Check sheet for the modelled part. Datum: model origin and axes. Units: mm. A direction names the side the tool comes from. Give positions to 0.01 mm unless a question says otherwise; leave off trailing zeros. Loops run counter-clockwise (first coordinate to the right, second up) from the corner with the lowest first, then second, coordinate; pieces in that order, holes last. Notation, with made-up numbers: M 54,-33 L 84,-33 A27 ccw 84,-8 Z; hole C -20,-33 d5. An arc over 180 degrees is marked long. Put each result on its own line as item: value. Start each with the question number.
```python
from build123d import *

# Parameters (mm, degrees)
SKETCH_1_R               = 23.95
EXTRUDE_1_DEPTH          = 1.25
SKETCH_2_W               = 2.45
SKETCH_2_H               = 4.95
CUT_EXTRUDE_1_DEPTH      = 3.5
SKETCH_3_R               = 0.75
CUT_EXTRUDE_2_DEPTH      = 3.5
SKETCH_4_R               = 1.55
CUT_EXTRUDE_3_DEPTH      = 3.5
PATTERN_CIRCULAR_1_COUNT = 5


with BuildPart() as part:
    # 草图1 → 凸台-拉伸1 (new body, symmetric)
    with BuildSketch(Plane.XY):
        with BuildLine():
            ThreePointArc((-15.121874884, 32.67), (-21.160269083, 29.124611797), (-26.398100061, 24.477342853))
            ThreePointArc((-26.398100061, 24.477342853), (-25.67852594, 8.343458848), (-35.743932713, -4.286172441))
            ThreePointArc((-35.743932713, -4.286172441), (-34.238034587, -11.124611797), (-31.43679796, -17.542170163))
            ThreePointArc((-31.43679796, -17.542170163), (-15.870201812, -21.843458848), (-6.969090425, -35.31900025))
            ThreePointArc((-6.969090425, -35.31900025), (0, -36), (6.969090425, -35.31900025))
            ThreePointArc((6.969090425, -35.31900025), (15.870201812, -21.843458848), (31.43679796, -17.542170163))
            ThreePointArc((31.43679796, -17.542170163), (34.238034587, -11.124611797), (35.743932713, -4.286172441))
            ThreePointArc((35.743932713, -4.286172441), (25.67852594, 8.343458848), (26.398100061, 24.477342853))
            ThreePointArc((26.398100061, 24.477342853), (21.160269083, 29.124611797), (15.121874884, 32.67))
            ThreePointArc((15.121874884, 32.67), (0, 27), (-15.121874884, 32.67))
        make_face()
        Circle(SKETCH_1_R, mode=Mode.SUBTRACT)
    extrude(amount=EXTRUDE_1_DEPTH, both=True)

    # 草图2 → 切除-拉伸1 (cut, through all)
    with BuildSketch(Plane.XY.offset(1.25)):
        with Locations((0, -31)):
            Rectangle(SKETCH_2_W, SKETCH_2_H)
    cut_extrude_1 = extrude(amount=-CUT_EXTRUDE_1_DEPTH, mode=Mode.SUBTRACT)

    # 草图3 → 切除-拉伸2 (cut, through all)
    with BuildSketch(Plane.XY.offset(1.25)):
        with Locations((-1.225, -29.275)):
            Circle(SKETCH_3_R)
        with Locations((1.225, -29.275)):
            Circle(SKETCH_3_R)
        with Locations((-1.225, -32.725)):
            Circle(SKETCH_3_R)
        with Locations((1.225, -32.725)):
            Circle(SKETCH_3_R)
    cut_extrude_2 = extrude(amount=-CUT_EXTRUDE_2_DEPTH, mode=Mode.SUBTRACT)

    # 草图4 → 切除-拉伸3 (cut, through all)
    with BuildSketch(Plane.XY.offset(1.25)):
        with Locations((-4.725, -30)):
            Circle(SKETCH_4_R)
        with Locations((4.725, -30)):
            Circle(SKETCH_4_R)
    cut_extrude_3 = extrude(amount=-CUT_EXTRUDE_3_DEPTH, mode=Mode.SUBTRACT)

    # 阵列(圆周)1: 切除-拉伸1, 切除-拉伸2, 切除-拉伸3 ×5 about axis
    pattern_circular_1_axis = Axis((0, 0, 0), (0, 0, 1))
    for i in range(1, PATTERN_CIRCULAR_1_COUNT):
        add(cut_extrude_1.rotate(pattern_circular_1_axis, i * 360 / PATTERN_CIRCULAR_1_COUNT), mode=Mode.SUBTRACT)
        add(cut_extrude_2.rotate(pattern_circular_1_axis, i * 360 / PATTERN_CIRCULAR_1_COUNT), mode=Mode.SUBTRACT)
        add(cut_extrude_3.rotate(pattern_circular_1_axis, i * 360 / PATTERN_CIRCULAR_1_COUNT), mode=Mode.SUBTRACT)


solid = part.part
```
Q1. Section check C-C, the plane z = 0.8. Give the number of separate pieces and of enclosed holes in the cut face, then the cut area to 3 significant figures.
Q2. Section check B-B, the plane y = 0. Record the cut outline in (x, z), then the cut area to 3 significant figures.
Q3. Thickness scan on line 1 along X through (y, z) = (-12.5, -0.5); line 2 along X through (y, z) = (26, -1.05); line 3 along Y through (x, z) = (13.5, 1.05). Record the ranges inside material, lowest first. Write a range as [from, to].
Q4. Section check A-A, the plane x = 0. Record the cut outline in (y, z) (3 decimals).
Q5. Mould release check, pull along Y, two halves, no side actions. Record for faces 3 (the face through (-11, -22, 1.25)), 4 (the face through (-31.535, -4.925, 0.018)), 5 (the face through (0, -36, 0)): pulls with the +Y half, pulls with the -Y half, needs draft (parallel to the pull), parting line crosses it, or undercut.
Q6. Access from +Z, -Z, +X, -X, +Y, -Y to the whole of each face (thin tool, end or side, straight path). Record for faces 1 (the face through (25.751, 8.124, 0.018)), 2 (the face through (29.874, -8.419, 0.018)).
Q7. Depth check by flat-ended pin: P1, Ø2.5, axis at x = 29.99, y = -4.78, coming from the -Z side; P2, Ø1, axis at y = -30.5, z = 0, coming from the +X side; P3, Ø0.6, axis at y = -30.5, z = 0.5, coming from the -X side; P4, Ø1.5, axis at y = 24.5, z = 1, coming from the +X side. Enter the tip coordinate at first touch or a pass-through.
Found:
1. separate pieces: 1
1. enclosed holes: 16
1. area: 1,190 mm^2
2. outline: M -30.52,-1.25 L -23.95,-1.25 L -23.95,1.25 L -30.52,1.25 Z; M 23.95,-1.25 L 30.52,-1.25 L 30.52,1.25 L 23.95,1.25 Z
2. area: 32.8 mm^2
3. line 1: x = [-33.76, -27.97], [-26.17, -20.43], [20.43, 26.17], [27.97, 33.76]
3. line 2: x = [-24.9, -20.94], [-17.38, -14.95], [-12.67, 12.67], [14.95, 17.38], [20.94, 24.9]
3. line 3: y = [-23.82, -19.78], [19.78, 25.53], [28.57, 31.38]
4. outline: M -36,-1.25 L -33.475,-1.25 L -33.475,1.25 L -36,1.25 Z; M -28.525,-1.25 L -23.95,-1.25 L -23.95,1.25 L -28.525,1.25 Z; M 23.95,-1.25 L 27,-1.25 L 27,1.25 L 23.95,1.25 Z
5. face 3: needs draft
5. face 4: undercut
5. face 5: pulls with the -Y half
6. face 1: +Z, -Z, +X
6. face 2: +Z, -Z
7. P1: passes through
7. P2: stops at x = 8.9
7. P3: stops at x = -8.8
7. P4: stops at x = 26.4
